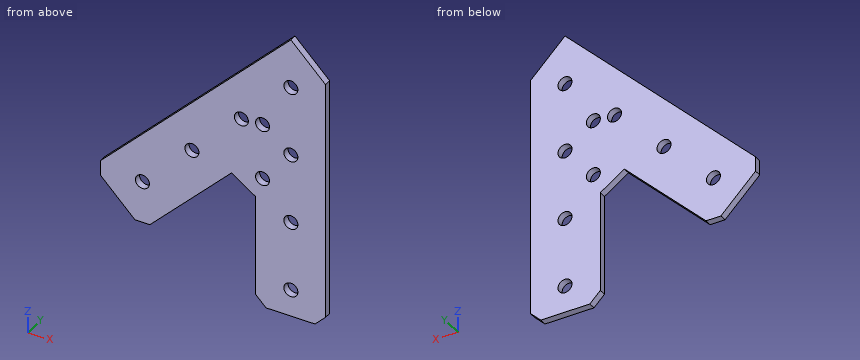
Autodesk Inventor part; units mm, degrees
ref_plane "YZ Plane" through (0, 0, 0) normal (1, 0, 0) x (0, 1, 0)
ref_plane "XZ Plane" through (0, 0, 0) normal (0, 1, 0) x (-1, 0, 0)
ref_plane "XY Plane" through (0, 0, 0) normal (0, 0, 1) x (1, 0, 0)
sketch "Sketch1" plane through (0, 0, 0) normal (0, 1, 0) x (-1, 0, 0)
  line L0 (0, 0) -> (12.5724, 12.5724)
  line L1 (0, 0) -> (17.78, 0) construction
  line L2 (25.4, -50.8) -> (34.125, -44.9013)
  circle A0 centre (66.4539, -59.2697) radius 2.54
  circle A1 centre (48.4934, -41.3092) radius 2.54
  circle A2 centre (30.5329, -23.3487) radius 2.54
  circle A3 centre (12.5724, -5.3882) radius 2.54
  circle A4 centre (12.5724, -30.7882) radius 2.54
  circle A5 centre (12.5724, -56.1882) radius 2.54
  circle A6 centre (12.5724, -81.5882) radius 2.54
  circle A7 centre (22.86, -43.18) radius 2.54
  circle A8 centre (22.86, -22.86) radius 2.54
  line L3 (81.7203, -56.5756) -> (81.7203, -61.9638)
  line L4 (69.148, -74.5361) -> (63.7598, -74.5361)
  line L5 (21.59, -91.44) -> (25.4, -87.63)
  line L6 (0, -87.63) -> (3.81, -91.44)
  line L7 (81.7203, -61.9638) -> (69.148, -74.5361)
  line L8 (81.7203, -56.5756) -> (12.5724, 12.5724)
  line L9 (0, 0) -> (0, -87.63)
  line L10 (3.81, -91.44) -> (21.59, -91.44)
  line L11 (25.4, -87.63) -> (25.4, -50.8)
  line L12 (34.125, -44.9013) -> (63.7598, -74.5361)
  dimension "d3" = 17.78
  dimension "d4" = 45
extrude "Extrusion1" add sketch "Sketch1" along normal blind 2.54
properties part number "1in 60deg bracket for alu extrusion" material "Steel, Alloy"
Read the model definition and answer for the solid it produces. Units are mm, in the model's axes. Round coordinates to 2 decimals unless told otherwise and drop trailing zeros. Order: outer loops, then holes, each group sorted by start corner. A loop starts at its lowest first (then second) coordinate and runs counter-clockwise, first axis right, second up.
1) The part is cut by section C-C on y = 1.8. Give the number of separate pieces and of enclosed holes in the cut face, plus the area to 3 significant figures.
2) The part is cut by section D-D on x = -6.5. Write down the section's boundary in (y, z), plus the area to 3 significant figures.
3) Straight lines are drawn through the part: L1, parallel to Z at x = -22.86, y = 1.1; L2, parallel to X at y = 0.6, z = -54; L3, parallel to X at y = 1.2, z = -32. For each, find the intervals that lie inside material, in ascending order.
4) The part is cut by section A-A on z = -65.5. Write down the section's boundary in (x, y).
5) Flat-ended cylindrical pins translate along their axes: pin 1 (8 mm diameter, centred on x = -66.45, z = -59.27, fed in from -Y); pin 2 (0.8 mm diameter, centred on x = -66.5, y = 1.5, fed in from -Z); pin 3 (1.5 mm diameter, centred on x = -32.5, y = 1.5, fed in from -Z); pin 4 (1.3 mm diameter, centred on y = 1.5, z = -73, fed in from -X). Find the tip coordinate at first contact, or state that the pin passes through.
6) The part is cut by section B-B on x = -22.86. Write down the section's boundary in (y, z).
Resolved:
1. separate pieces: 1
1. enclosed holes: 9
1. area: 4,130 mm2
2. outline: (0, -91.44) - (2.54, -91.44) - (2.54, 6.5) - (0, 6.5) - close
2. area: 249 mm2
3. L1: z = -90.17 to -45.72, -40.64 to -25.4, -20.32 to 2.28
3. L2: x = -79.14 to -43.22, -25.4 to -13.86, -11.28 to 0
3. L3: x = -57.14 to -14.8, -10.34 to 0
4. outline: (-78.18, 0) - (-54.72, 0) - (-54.72, 2.54) - (-78.18, 2.54) - close; (-25.4, 0) - (0, 0) - (0, 2.54) - (-25.4, 2.54) - close
5. pin 1: stops at y = 0
5. pin 2: stops at z = -74.54
5. pin 3: stops at z = -46.51
5. pin 4: stops at x = -71.33
6. outline: (0, -90.17) - (2.54, -90.17) - (2.54, -45.72) - (0, -45.72) - close; (0, -40.64) - (2.54, -40.64) - (2.54, -25.4) - (0, -25.4) - close; (0, -20.32) - (2.54, -20.32) - (2.54, 2.28) - (0, 2.28) - close
